```python
from build123d import *

# Parameters (mm, degrees)
BOSS_EXTRUDE1_DEPTH   = 9.525
SKETCH4_R             = 6.35
SKETCH4_W             = 25.4
SKETCH4_H             = 3.175
BOSS_EXTRUDE2_DEPTH   = 9.525
F_6_CLEARANCE_HOLE1_D = 3.7973
F_6_CLEARANCE_HOLE2_D = 3.7973


with BuildPart() as part:
    # Sketch1 → Boss-Extrude1 (new body)
    with BuildSketch(Plane.XY):
        with BuildLine():
            Line((11.8364, 8.1026), (-0.896679191, 6.286371483))
            ThreePointArc((-0.896679191, 6.286371483), (-6.286371483, -0.896679191), (0.896679191, -6.286371483))
            Line((0.896679191, -6.286371483), (37.2364, -1.102924791))
            Line((37.2364, -1.102924791), (37.2364, 8.1026))
            Line((37.2364, 8.1026), (11.8364, 8.1026))
        make_face()
    extrude(amount=BOSS_EXTRUDE1_DEPTH)

    # Sketch4 → Boss-Extrude2 (add)
    with BuildSketch(Plane.XY.offset(9.525)):
        with Locations(Location((0, 0, 0), (0, 0, 98.117830505))):
            Circle(SKETCH4_R)
        with Locations((24.5364, 6.5151)):
            Rectangle(SKETCH4_W, SKETCH4_H)
    extrude(amount=BOSS_EXTRUDE2_DEPTH)

    # #6 Clearance Hole1 (through all)
    with Locations(Plane(origin=(0, 0, 0), x_dir=(-1, 0, 0), z_dir=(0, 0, -1))):
        with Locations((0, 0)):
            Hole(F_6_CLEARANCE_HOLE1_D / 2)

    # #6 Clearance Hole2 (through all)
    with Locations(Plane(origin=(16.7894, 4.9276, 14.2875), x_dir=(-1, 0, 0), z_dir=(0, -1, 0))):
        with Locations((0, 0), (-12.7, 0)):
            Hole(F_6_CLEARANCE_HOLE2_D / 2)


solid = part.part
```
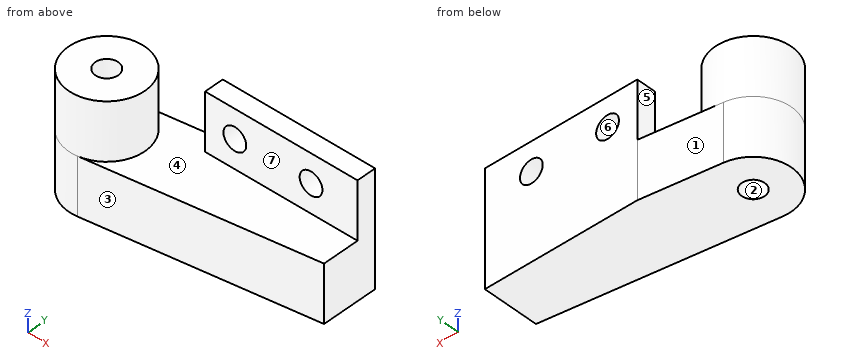
Check sheet for the modelled part. Datum: model origin and axes. Units: mm. Face numbers are marked on the shaded views. A direction names the side the tool comes from. Coordinates: 2 decimals unless noted, no trailing zeros. Order: outer loops, then holes, each group sorted by start corner. A loop starts at its lowest first (then second) coordinate and runs counter-clockwise, first axis right, second up. Notation, with made-up numbers: (-1, 42) -> (43, 42) arc R18 cw to (43, 70) -> close; hole circle Ø8 at (20.25, -16.5). An arc over 180 degrees is marked (long way). Write item = value, one per line. Start each with the question number.
1) Mould release check, pull along Y, two halves, no side actions. Record for the marked faces 1, 2, 3 and 4: +Y half, -Y half, draft (parallel to the pull), parting line (faces both ways), or undercut.
2) Cross-section at C-C (x = 0). Enter the section's corners in (y, z) (3 decimals).
3) Cross-section at B-B (z = 3.25). Enter the section's corners in (x, y).
4) Go/stop test with flat-tipped pins: P1, Ø10.5, axis at x = 27, z = 14, coming from the -Y side; P2, Ø1, axis at x = 18, z = 13, coming from the -Y side; P3, Ø4, axis at y = 0.5, z = 16, coming from the +X side. Record where each tip stops, or that it passes through.
5) Cross-section at D-D (x = 25). Enter the section's corners in (y, z) (3 decimals).
6) Material ranges on L1, parallel to Y at x = 1, z = 8; L2, parallel to Y at x = 0, z = 7.25; L3, parallel to Z at x = 23, y = 2.75 (3 decimals), recorded low to high.
7) Access from +Z, -Z, +X, -X, +Y, -Y to the whole of each face (thin tool, end or side, straight path). Record for the marked faces 5, 6 and 7.
8) Cross-section at A-A (y = 0). Enter the section's corners in (x, z) (3 decimals).
Ans:
q1.face_1 = +Y half
q1.face_2 = undercut
q1.face_3 = -Y half
q1.face_4 = draft
q2.outline = (-6.35, 0) -> (-1.899, 0) -> (-1.899, 19.05) -> (-6.35, 19.05) -> close; (1.899, 0) -> (6.414, 0) -> (6.414, 9.525) -> (6.35, 9.525) -> (6.35, 19.05) -> (1.899, 19.05) -> close
q3.outline = (-0.9, 6.29) arc R6.35 ccw to (0.9, -6.29) -> (37.24, -1.1) -> (37.24, 8.1) -> (11.84, 8.1) -> close; hole circle Ø3.8 at (0, 0)
q4.P1 = -2.95
q4.P2 = 4.93
q4.P3 = 6.35
q5.outline = (-2.848, 0) -> (8.103, 0) -> (8.103, 19.05) -> (4.928, 19.05) -> (4.928, 9.525) -> (-2.848, 9.525) -> close
q6.L1 = -6.27 to -1.61, 1.61 to 6.56
q6.L2 = -6.35 to -1.9, 1.9 to 6.41
q6.L3 = 0 to 9.525
q7.face_5 = +Z, +Y, -Y
q7.face_6 = +Y, -Y
q7.face_7 = +Z, +X, -Y
q8.outline = (-6.35, 0) -> (-1.899, 0) -> (-1.899, 19.05) -> (-6.35, 19.05) -> close; (1.899, 0) -> (37.236, 0) -> (37.236, 9.525) -> (6.35, 9.525) -> (6.35, 19.05) -> (1.899, 19.05) -> close
